from build123d import *

# Parameters (mm, degrees)
CYLINDER023_R     = 1.8
CYLINDER023_DEPTH = 40
ARRAY002_Z_COUNT  = 3
ARRAY002_Z_PITCH  = 15
BOX_W             = 14
BOX_H             = 4
BOX_DEPTH         = 55
FILLET003_R       = 10


with BuildPart() as attachment_hole_array:
    # Cylinder023 → Cylinder023 (new body)
    with BuildSketch(Plane(origin=(19, -20, 0), x_dir=(1, 0, 0), z_dir=(0, 1, 0))):
        Circle(CYLINDER023_R)
    extrude(amount=CYLINDER023_DEPTH)

    # Array002 Z: attachment hole array ×3


with BuildPart() as attachment_hole_array_1:
    add(attachment_hole_array.part)
    with Locations(*[(0, 0, i * ARRAY002_Z_PITCH) for i in range(1, ARRAY002_Z_COUNT)]):
        add(attachment_hole_array.part)


with BuildPart() as attachment_hole_array_2:
    # Array002 placement: moved
    add(attachment_hole_array_1.part.moved(Location((0, 0, 15))))


with BuildPart() as attachment_cut:
    # Box → Box (new body)
    with BuildSketch(Plane(origin=(12, -2, 0), x_dir=(1, 0, 0), z_dir=(0, 0, 1))):
        with Locations((7, 2)):
            Rectangle(BOX_W, BOX_H)
    extrude(amount=BOX_DEPTH)

    # Fillet003
    fillet003_edges = [attachment_cut.edges().sort_by_distance(p)[0] for p in [
        (26, 0, 55),
        (26, 0, 0),
    ]]
    fillet(fillet003_edges, radius=FILLET003_R)

    # Cut004: cut attachment hole array
    add(attachment_hole_array_2.part, mode=Mode.SUBTRACT)


with BuildPart() as attachment_cut_1:
    # Cut004 placement: moved
    add(attachment_cut.part.moved(Location((0, 0, 4))))


solid = attachment_cut_1.part
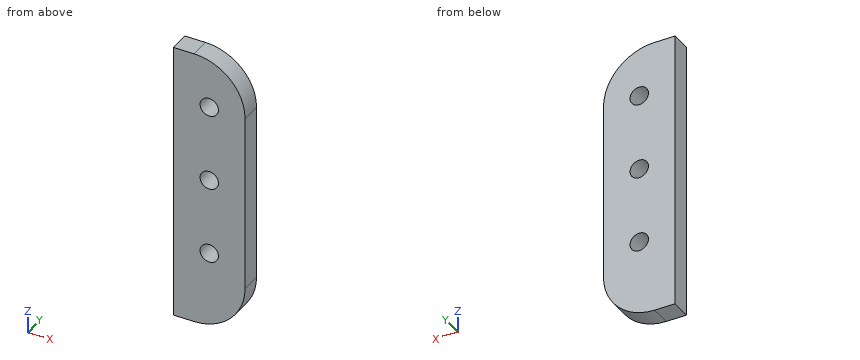
Check sheet for the modelled part. Datum: model origin and axes. Units: mm. Round coordinates to 2 decimals unless told otherwise and drop trailing zeros. Loops run counter-clockwise (first coordinate to the right, second up) from the corner with the lowest first, then second, coordinate; pieces in that order, holes last. Notation, with made-up numbers: M 72.5,-39.5 L 104.5,-39.5 A31 ccw 104.5,-11.5 Z; hole C -10.5,-30.5 d7. An arc over 180 degrees is marked long. One line per question, with ' | ' between items. Start each with the question number.
Item 1: Section check D-D (z = 49.5). Record the boundary of the cut face in (x, y), and give its area (3 significant figures).
Item 2: Section check C-C (x = 18). Record the boundary of the cut face in (y, z), and give its area (3 significant figures).
Item 3: Scan lines: probe 1 along Z at (x, y) = (19, 1.15); probe 2 along Z at (x, y) = (20.5, -1.65); probe 3 along X at (y, z) = (1.8, 34.5). Record each from-to range of solid material in increasing order.
Item 4: Section check B-B (z = 19). Record the boundary of the cut face in (x, y), and give its area (3 significant figures).
Item 5: Section check A-A (y = -0.35). Record the boundary of the cut face in (x, z).
Item 6: Gauge pin test, flat ends, axial feed: pin 1 Ø3 at (x, z) = (19, 34) entering from +Y; pin 2 Ø4 at (x, z) = (19, 49) entering from +Y; pin 3 Ø1 at (x, y) = (24, 0) entering from -Z; pin 4 Ø2 at (x, y) = (18.5, 0.5) entering from +Z. Record the tip position at first contact, or that the pin passes through.
Worked out:
1) outline: M 12,-2 L 17.27,-2 L 17.27,2 L 12,2 Z; M 20.73,-2 L 25.99,-2 L 25.99,2 L 20.73,2 Z | area: 42.1 mm^2
2) outline: M -2,4.2 L 2,4.2 L 2,17.5 L -2,17.5 Z; M -2,20.5 L 2,20.5 L 2,32.5 L -2,32.5 Z; M -2,35.5 L 2,35.5 L 2,47.5 L -2,47.5 Z; M -2,50.5 L 2,50.5 L 2,58.8 L -2,58.8 Z | area: 182 mm^2
3) probe 1: 4.46 to 17.2, 20.8 to 32.2, 35.8 to 47.2, 50.8 to 58.54 | probe 2: 5.07 to 18.01, 19.99 to 33.01, 34.99 to 48.01, 49.99 to 57.93 | probe 3: 12 to 17.27, 20.73 to 26
4) outline: M 12,-2 L 17.2,-2 L 17.2,2 L 12,2 Z; M 20.8,-2 L 26,-2 L 26,2 L 20.8,2 Z | area: 41.6 mm^2
5) outline: M 12,4 L 16,4 A10 ccw 26,14 L 26,49 A10 ccw 16,59 L 12,59 Z; hole C 19,19 d3.6; hole C 19,34 d3.6; hole C 19,49 d3.6
6) pin 1: through | pin 2: y = 2 | pin 3: z = 7.39 | pin 4: z = 58.89
